Input: dimensioned drawing with shaded views. Units: mm. Origin: part minimum x, y, z. A direction names the side the tool comes from. Round coordinates to 2 decimals unless told otherwise and drop trailing zeros. Order: outer loops, then holes, each group sorted by start corner. A loop starts at its lowest first (then second) coordinate and runs counter-clockwise, first axis right, second up. Notation, with made-up numbers: M 34.25,57 L 50.25,57 A13 ccw 50.25,70 Z; hole C 65,72 d5. An arc over 180 degrees is marked long. Use one line per item in the form item = value. Start each with the question number.
Q1. Section B-B (x = 21.5). Return the cut outline in (y, z), plus the area to 3 significant figures.
Q2. Section C-C (z = 42). Return the cut outline in (x, y).
Q3. Material intervals for probe 1 along Y at (x, z) = (23, 42); probe 2 along Z at (x, y) = (26, 4.75); probe 3 along Z at (x, y) = (36.5, 5.25), sorted ascending.
Q4. Pull-direction query (X, two-part tool) for the marked faces 6, 7, 8 and 9; classes: pulls with the +X half, pulls with the -X half, needs draft (parallel to the pull), parting line crosses it, or undercut.
Q5. Section A-A (y = 2.5). Return the cut outline in (x, z).
Q6. Section D-D (x = 39). Return the cut outline in (y, z), plus the area to 3 significant figures.
Q7. Reachability of the marked faces 1, 2, 3, 4 and 5 from +Z, -Z, +X, -X, +Y, -Y: full face, straight path, thin tool, end or side. Return the list, or none.
Q8. Contact query for flat-ended pins moving along their axis: pin 1 (4 mm diameter, centred on y = 3, z = 38, fed in from +X); pin 2 (4 mm diameter, centred on x = 40.5, y = 2.5, fed in from +Z); pin 3 (3 mm diameter, centred on x = 25, y = 7, fed in from +Z); pin 4 (3.5 mm diameter, centred on x = 6.5, z = 4, fed in from +Y). Output: stop coordinate, or through.
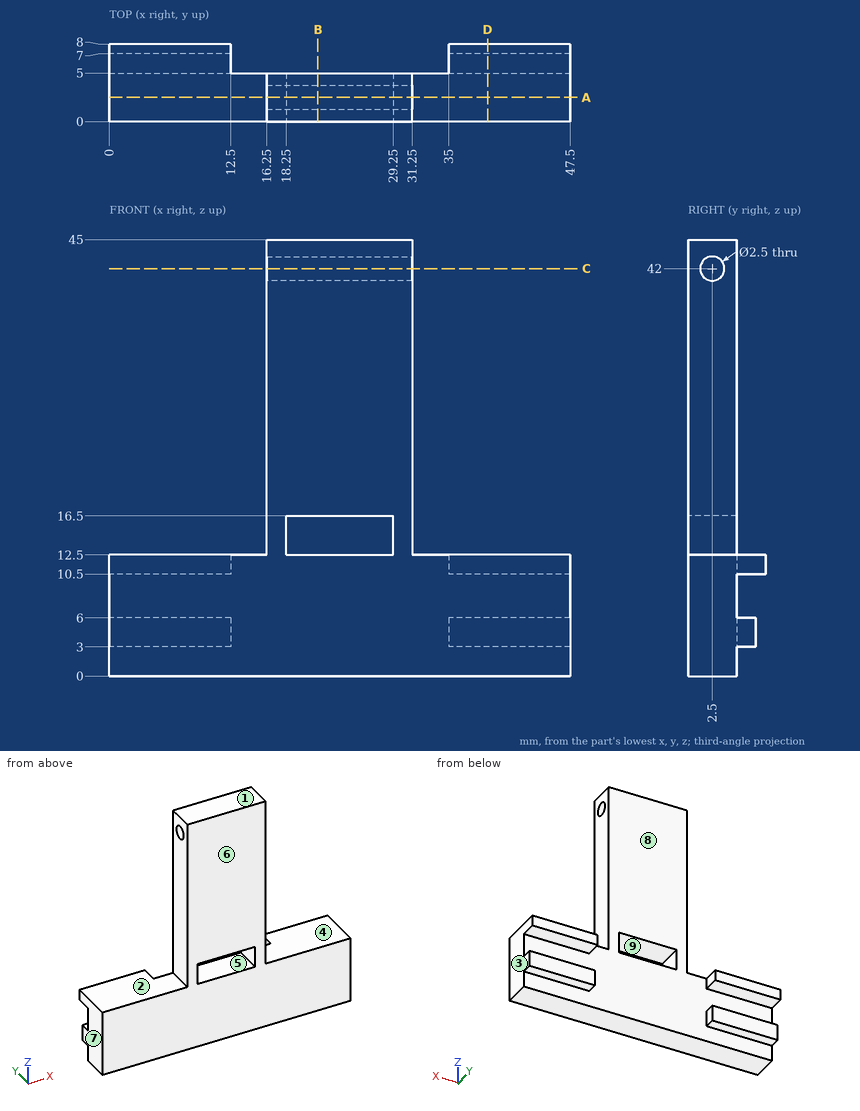
Results list:
q1.outline = M 0,0 L 5,0 L 5,12.5 L 0,12.5 Z; M 0,16.5 L 5,16.5 L 5,45 L 0,45 Z; hole C 2.5,42 d2.5
q1.area = 200 mm2
q2.outline = M 16.25,0 L 31.25,0 L 31.25,1.25 L 16.25,1.25 Z; M 16.25,3.75 L 31.25,3.75 L 31.25,5 L 16.25,5 Z
q3.probe_1 = 0 to 1.25, 3.75 to 5
q3.probe_2 = 0 to 12.5, 16.5 to 45
q3.probe_3 = 3 to 6, 10.5 to 12.5
q4.face_6 = needs draft
q4.face_7 = pulls with the -X half
q4.face_8 = undercut
q4.face_9 = undercut
q5.outline = M 0,0 L 47.5,0 L 47.5,12.5 L 31.25,12.5 L 31.25,40.75 L 16.25,40.75 L 16.25,12.5 L 0,12.5 Z; M 16.25,43.25 L 31.25,43.25 L 31.25,45 L 16.25,45 Z; hole M 18.25,12.5 L 29.25,12.5 L 29.25,16.5 L 18.25,16.5 Z
q6.outline = M 0,0 L 5,0 L 5,3 L 7,3 L 7,6 L 5,6 L 5,10.5 L 8,10.5 L 8,12.5 L 0,12.5 Z
q6.area = 74.5 mm2
q7.face_1 = +Z, +X, -X, +Y, -Y
q7.face_2 = +Z, -X, +Y, -Y
q7.face_3 = +Z, -Z, +X, +Y, -Y
q7.face_4 = +Z, +X, +Y, -Y
q7.face_5 = +Y, -Y
q8.pin_1 = 31.25
q8.pin_2 = 12.5
q8.pin_3 = through
q8.pin_4 = 7
